Work out the finished part from the listing and answer in its coordinate system (mm). A direction names the side the tool comes from. Round coordinates to 2 decimals unless told otherwise and drop trailing zeros. Write each loop counter-clockwise with the first axis right and the second up, starting at its lowest first coordinate (ties: lowest second). Pieces come first, ordered by that corner, then holes.
1. Find section A-A (x = 0). Write down the section's boundary in (y, z), and give its area (3 significant figures).
2. Flat-ended cylindrical pins translate along their axes: pin 1 Ø5 at (x, y) = (10.5, 17) entering from +Z; pin 2 Ø1 at (y, z) = (-7.5, 17) entering from +X; pin 3 Ø3 at (y, z) = (3, 9.5) entering from +X. Find the tip coordinate at first contact, or state that the pin passes through.
3. Straight lines are drawn through the part: probe 1 along Z at (x, y) = (5, 14); probe 2 along Y at (x, z) = (0, 16.5); probe 3 along Y at (x, z) = (0, 13). For each, find the intervals that lie inside material, in ascending order.
4. Determine the mould class of faces 4 (the face through (3, 0, 10)), 5 (the face through (-0.2, -3.5, 21.2)), 6 (the face through (-1.269, -9.667, 13.071)) for opening direction Y: pulls with the +Y half, pulls with the -Y half, needs draft (parallel to the pull), parting line crosses it, or undercut.
5. A tool of negligible diameter and unlimited length cuts with its end or side. For faces 1 (the face through (-6.4, 17.3, 3)), 2 (the face through (4, 0, 0)), 3 (the face through (8, -8, 15.2)), from which of +Z, -Z, +X, -X, +Y, -Y can it reach the whole face along a straight path? Write none if from no direction.
Autodesk Inventor part; units mm, degrees
ref_plane "YZ Plane" through (0, 0, 0) normal (1, 0, 0) x (0, 1, 0)
ref_plane "XZ Plane" through (0, 0, 0) normal (0, 1, 0) x (-1, 0, 0)
ref_plane "XY Plane" through (0, 0, 0) normal (0, 0, 1) x (1, 0, 0)
sketch "Skizze1" plane through (0, 0, 0) normal (0, 0, 1) x (1, 0, 0)
  circle A0 centre (0, 0) radius 21.1
  dimension "d0" = 42.2
extrude "Extrusion1" add sketch "Skizze1" along normal blind 3
sketch "Skizze2" plane through (0, 0, 3) normal (0, 0, 1) x (1, 0, 0)
  circle A0 centre (0, 0) radius 18.25
  dimension "d3" = 36.5
extrude "Extrusion2" add sketch "Skizze2" along normal blind 8
sketch "Skizze3" plane through (0, 0, 11) normal (0, 0, 1) x (1, 0, 0)
  circle A0 centre (0, 0) radius 9.75
  dimension "d6" = 19.5
extrude "Extrusion3" add sketch "Skizze3" along normal blind 4.2
sketch "Skizze4" plane through (0, 0, 15.2) normal (0, 0, 1) x (1, 0, 0)
  circle A0 centre (0, 0) radius 18.25
  dimension "d12" = 36.5
extrude "Extrusion4" add sketch "Skizze4" along normal blind 6
fillet "Rundung1" radius 1.5 1 edges at (-18.25, 0, 21.2)
sketch "Skizze5" plane through (0, 0, 0) normal (0, 0, -1) x (-1, 0, 0)
  circle A0 centre (0, 0) radius 3
  dimension "d13" = 6
extrude "Extrusion5" cut sketch "Skizze5" against normal blind 100
properties part number "Pfropfen_mittel"
Worked answers:
1. outline: (-21.1, 0) - (-3, 0) - (-3, 21.2) - (-16.75, 21.2) arc R1.5 ccw to (-18.25, 19.7) - (-18.25, 15.2) - (-9.75, 15.2) - (-9.75, 11) - (-18.25, 11) - (-18.25, 3) - (-21.1, 3) - close; (3, 0) - (21.1, 0) - (21.1, 3) - (18.25, 3) - (18.25, 11) - (9.75, 11) - (9.75, 15.2) - (18.25, 15.2) - (18.25, 19.7) arc R1.5 ccw to (16.75, 21.2) - (3, 21.2) - close
1. area: 591 mm2
2. pin 1: stops at z = 21.01
2. pin 2: stops at x = 16.85
2. pin 3: stops at x = 18.19
3. probe 1: z = 0 to 11, 15.2 to 21.2
3. probe 2: y = -18.25 to -3, 3 to 18.25
3. probe 3: y = -9.75 to -3, 3 to 9.75
4. face 4: undercut
4. face 5: needs draft
4. face 6: parting line crosses it
5. face 1: +Z
5. face 2: -Z, +X, -X, +Y, -Y
5. face 3: none
